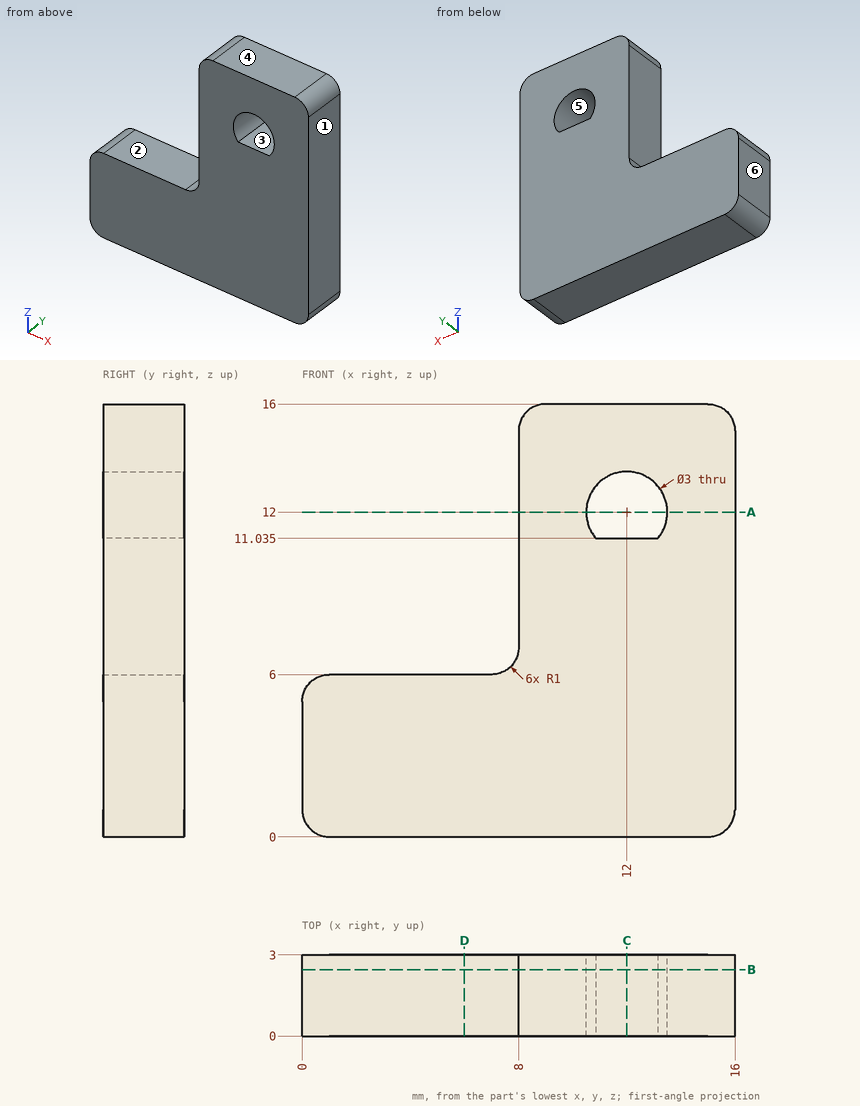
Part print with two shaded views. Sizes in mm from the minimum x, y, z corner. A direction names the side the tool comes from. Round coordinates to 2 decimals unless told otherwise and drop trailing zeros. Loops run counter-clockwise (first coordinate to the right, second up) from the corner with the lowest first, then second, coordinate; pieces in that order, holes last. Notation, with made-up numbers: M 57,10 L 90,10 A17 cw 90,37 Z; hole C -22,31.25 d5. An arc over 180 degrees is marked long. Put each result on its own line as item: value. Start each with the question number.
Item 1: Drop flat-ended pins along their axis: P1, Ø1, axis at y = 1, z = 11.5, coming from the -X side; P2, Ø1.5, axis at y = 0.5, z = 7, coming from the -X side; P3, Ø1.5, axis at x = 6.5, y = 1.5, coming from the +Z side. Give the stop position or say it passes through.
Item 2: Cut at B-B (y = 2.45). List the corners of the cut face in (x, z) (1 decimal).
Item 3: Cut at A-A (z = 12). List the corners of the cut face in (x, y), then the cut area to 3 significant figures.
Item 4: Mould opens along Z. For the marked faces 4, 5 and 6 say: released by +Z, released by -Z, zero draft, split by the parting line, or undercut.
Item 5: Cut at C-C (x = 12). List the corners of the cut face in (y, z) (1 decimal), then the cut area to 3 significant figures.
Item 6: 3-axis set-ups, long thin cutter, end or side, ignore diameter. For the marked faces 1, 2 and 3: which of +Z, -Z, +X, -X, +Y, -Y reach the whole face in a straight line?
Item 7: Cut at D-D (x = 6). List the corners of the cut face in (y, z).
Item 8: Drill centre lines: line 1 along Z through (x, y) = (12, 0.95) (1 decimal); line 2 along X through (y, z) = (2.15, 12); line 3 along X through (y, z) = (1.65, 10.25). Where is each one in solid material? Low to high.
Answer block:
1. P1: x = 8
1. P2: x = 7.66
1. P3: z = 6.03
2. outline: M 0,1 A1 ccw 1,0 L 15,0 A1 ccw 16,1 L 16,15 A1 ccw 15,16 L 9,16 A1 ccw 8,15 L 8,7 A1 cw 7,6 L 1,6 A1 ccw 0,5 Z; hole M 10.9,11 L 13.1,11 A1.5 ccw long Z
3. outline: M 8,0 L 10.5,0 L 10.5,3 L 8,3 Z; M 13.5,0 L 16,0 L 16,3 L 13.5,3 Z
3. area: 15.0 mm2
4. face 4: released by +Z
4. face 5: undercut
4. face 6: zero draft
5. outline: M 0,0 L 3,0 L 3,11 L 0,11 Z; M 0,13.5 L 3,13.5 L 3,16 L 0,16 Z
5. area: 40.6 mm2
6. face 1: +Z, -Z, +X, +Y, -Y
6. face 2: +Z, -X, +Y, -Y
6. face 3: +Y, -Y
7. outline: M 0,0 L 3,0 L 3,6 L 0,6 Z
8. line 1: 0 to 11, 13.5 to 16
8. line 2: 8 to 10.5, 13.5 to 16
8. line 3: 8 to 16
